from build123d import *

# Parameters (mm, degrees)
F0_R      = 5.334
F1_DEPTH  = 37.084
F2_R      = 2.032
F3_DEPTH  = 8.128
F4_W      = 3.0226
F4_H      = 47.752
F5_DEPTH  = 10.16
F7_DEPTH  = 3.0226
F9_DEPTH  = 3.0226
F10_R     = 2.54
F11_R     = 1.143
F13_DEPTH = 0.127


# Not quite as in the source:
# - a feature of the source that left no trace in its solid (it failed there, or was rolled back) is left out


with BuildPart() as f1:
    # F0 (on Top) → F1 (new body)
    with BuildSketch(Plane.XY):
        Circle(F0_R)
    extrude(amount=F1_DEPTH)

    # F2 (on Front) → F3 (join)
    with BuildSketch(Plane.XZ):
        with Locations((0, 6.2738)):
            Circle(F2_R)
    extrude(amount=-F3_DEPTH)

    # F4 (on face) → F5 (join, symmetric)
    with BuildSketch(Plane.XY.offset(37.084)):
        with Locations((0, 13.208)):
            Rectangle(F4_W, F4_H)
    extrude(amount=F5_DEPTH, both=True)

    # F6 (on face) → F7 (join)
    with BuildSketch(Plane(origin=(-1.5113, 0, 0), x_dir=(0, -1, 0), z_dir=(-1, 0, 0))):
        Polygon((15.748, 47.244), (10.668, 47.244), (10.668, 26.924), align=None)
        Polygon((-37.084, 47.244), (-37.084, 26.924), (-32.004, 47.244), align=None)
    extrude(amount=-F7_DEPTH)

    # F8 (on face) → F9 (cut, through all)
    with BuildSketch(Plane(origin=(-1.5113, 0, 0), x_dir=(0, -1, 0), z_dir=(-1, 0, 0))):
        Polygon((-37.084, 47.244), (-37.084, 26.924), (-32.004, 47.244), align=None)
    extrude(amount=-F9_DEPTH, mode=Mode.SUBTRACT)

    # F10
    f10_edges = [f1.edges().sort_by_distance(p)[0] for p in [
        (0, 32.004, 47.244),
        (0, 37.084, 26.924),
        (0, -15.748, 47.244),
        (0, -10.668, 26.924),
    ]]
    fillet(f10_edges, radius=F10_R)

    # F11
    f11_edges = [f1.edges().sort_by_distance(p)[0] for p in [
        (-1.5113, 8.763, 47.244),
        (1.5113, 8.763, 47.244),
        (-1.5113, 34.38999, 37.70004),
        (1.5113, 34.38999, 37.70004),
        (1.5113, 31.583975, 46.706042),
        (-1.5113, 31.583975, 46.706042),
        (-1.5113, 35.83287, 27.900853),
        (1.5113, 35.83287, 27.900853),
        (1.5113, 19.473124, 26.924),
        (-1.5113, 19.473124, 26.924),
        (1.5113, -14.49687, 46.267147),
        (1.5113, -13.05399, 36.46796),
        (-1.5113, -14.49687, 46.267147),
        (-1.5113, -13.05399, 36.46796),
        (1.5113, -10.247975, 27.461958),
        (1.5113, -6.900124, 26.924),
        (-1.5113, -6.900124, 26.924),
        (-1.5113, -10.247975, 27.461958),
    ]]
    fillet(f11_edges, radius=F11_R)

    # F12 (on face) → F13 (join)
    with BuildSketch(Plane.YZ.offset(1.5113)):
        with BuildLine():
            Line((-6.1186332318, 29.319293674), (-9.2636532318, 29.319293674))
            ThreePointArc((-9.2636532318, 29.319293674), (-9.0520071402, 28.9937255277), (-8.6848279277, 28.8673605332))
            Line((-8.6848279277, 28.8673605332), (-5.9157811718, 28.8673605332))
            Line((-5.9157811718, 28.8673605332), (-6.1186332318, 29.319293674))
        make_face()
        Polygon((-9.9286332318, 44.559293674), (-13.0736532318, 44.559293674), (-9.2636532318, 29.319293674), (-6.1186332318, 29.319293674), align=None)
        Polygon((-3.6385932318, 44.559293674), (-6.7836132318, 44.559293674), (-5.1148799466, 37.8843605332), (-1.9698599466, 37.8843605332), align=None)
        Polygon((2.6514467682, 44.559293674), (-0.4935732318, 44.559293674), (1.1751600534, 37.8843605332), (4.3201800534, 37.8843605332), align=None)
        with BuildLine():
            ThreePointArc((33.8308279277, 28.8673605332), (34.3011024, 29.0968207875), (34.4096532318, 29.608706326))
            Line((34.4096532318, 29.608706326), (33.8308279277, 29.464))
            Line((33.8308279277, 29.464), (31.6216067682, 29.319293674))
            Line((31.6216067682, 29.319293674), (28.4765867682, 29.319293674))
            Line((28.4765867682, 29.319293674), (25.3315667682, 29.319293674))
            Line((25.3315667682, 29.319293674), (22.1865467682, 29.319293674))
            Line((22.1865467682, 29.319293674), (19.0415267682, 29.319293674))
            Line((19.0415267682, 29.319293674), (15.8965067682, 29.319293674))
            Line((15.8965067682, 29.319293674), (12.7514867682, 29.319293674))
            Line((12.7514867682, 29.319293674), (9.6064667682, 29.319293674))
            Line((9.6064667682, 29.319293674), (6.4614467682, 29.319293674))
            Line((6.4614467682, 29.319293674), (5.9157811718, 31.5019560598))
            Line((5.9157811718, 31.5019560598), (5.9157811718, 28.8673605332))
            Line((5.9157811718, 28.8673605332), (33.8308279277, 28.8673605332))
        make_face()
        with BuildLine():
            ThreePointArc((-12.4948279277, 45.3006394668), (-12.9651024, 45.0711792125), (-13.0736532318, 44.559293674))
            Line((-13.0736532318, 44.559293674), (-9.9286332318, 44.559293674))
            Line((-9.9286332318, 44.559293674), (-6.7836132318, 44.559293674))
            Line((-6.7836132318, 44.559293674), (-3.6385932318, 44.559293674))
            Line((-3.6385932318, 44.559293674), (-0.4935732318, 44.559293674))
            Line((-0.4935732318, 44.559293674), (2.6514467682, 44.559293674))
            Line((2.6514467682, 44.559293674), (5.7964667682, 44.559293674))
            Line((5.7964667682, 44.559293674), (8.9414867682, 44.559293674))
            Line((8.9414867682, 44.559293674), (12.0865067682, 44.559293674))
            Line((12.0865067682, 44.559293674), (15.2315267682, 44.559293674))
            Line((15.2315267682, 44.559293674), (18.3765467682, 44.559293674))
            Line((18.3765467682, 44.559293674), (21.5215667682, 44.559293674))
            Line((21.5215667682, 44.559293674), (24.6665867682, 44.559293674))
            Line((24.6665867682, 44.559293674), (27.8116067682, 44.559293674))
            Line((27.8116067682, 44.559293674), (30.6720063948, 44.559293674))
            Line((30.6720063948, 44.559293674), (30.5996532318, 44.848706326))
            ThreePointArc((30.5996532318, 44.848706326), (30.3880071402, 45.1742744723), (30.0208279277, 45.3006394668))
            Line((30.0208279277, 45.3006394668), (-12.4948279277, 45.3006394668))
        make_face()
        Polygon((8.9414867682, 44.559293674), (5.7964667682, 44.559293674), (9.6064667682, 29.319293674), (12.7514867682, 29.319293674), align=None)
        Polygon((15.2315267682, 44.559293674), (12.0865067682, 44.559293674), (15.8965067682, 29.319293674), (19.0415267682, 29.319293674), align=None)
        Polygon((25.3315667682, 29.319293674), (21.5215667682, 44.559293674), (18.3765467682, 44.559293674), (22.1865467682, 29.319293674), align=None)
        Polygon((31.6216067682, 29.319293674), (27.8116067682, 44.559293674), (24.6665867682, 44.559293674), (28.4765867682, 29.319293674), align=None)
    extrude(amount=F13_DEPTH)

    # F14: F1 across plane


with BuildPart() as f1_1:
    add(f1.part)
    add(f1.part.mirror(Plane.YZ))

    # F17: F1 across plane


with BuildPart() as f1_2:
    add(f1_1.part)
    add(f1_1.part.mirror(Plane.YZ))


solid = f1_2.part
Could you check a few things on this model? Use its own coordinates, in mm. A direction names the side the tool comes from. Round coordinates to 2 decimals unless told otherwise and drop trailing zeros. Order: outer loops, then holes, each group sorted by start corner. A loop starts at its lowest first (then second) coordinate and runs counter-clockwise, first axis right, second up. Notation, with made-up numbers: M -1.75,-7 L 38.25,-7 A26 ccw 38.25,22 Z; hole C 6,35 d2. An arc over 180 degrees is marked long. One line per item, written item: value.
(1) Imagine slicing it at C-C (y = -4.5). Write out the boundary of the cut face in (x, z), and give its area (3 significant figures).
Ans:
outline: M -2.86,0 L 2.86,0 L 2.86,37.08 L 1.51,37.08 L 1.51,37.88 L 1.64,37.88 L 1.64,45.3 L 1.51,45.3 L 1.51,46.1 A1.14 ccw 0.37,47.24 L -0.37,47.24 A1.14 ccw -1.51,46.1 L -1.51,45.3 L -1.64,45.3 L -1.64,37.88 L -1.51,37.88 L -1.51,37.08 L -2.86,37.08 Z
area: 244 mm^2
(2) Imagine slicing it at D-D (x = -4.25). Write out the boundary of the cut face in (y, z), and give its area (3 significant figures).
Ans:
outline: M -3.22,0 L 3.22,0 L 3.22,37.08 L -3.22,37.08 Z
area: 239 mm^2
(3) Imagine slicing it at A-A (y = 27). Write out the boundary of the cut face in (x, z), and give its area (3 significant figures).
Ans:
outline: M -1.64,28.87 L -1.51,28.87 L -1.51,28.07 A1.14 ccw -0.37,26.92 L 0.37,26.92 A1.14 ccw 1.51,28.07 L 1.51,28.87 L 1.64,28.87 L 1.64,29.32 L 1.51,29.32 L 1.51,35.23 L 1.64,35.23 L 1.64,45.3 L 1.51,45.3 L 1.51,46.1 A1.14 ccw 0.37,47.24 L -0.37,47.24 A1.14 ccw -1.51,46.1 L -1.51,45.3 L -1.64,45.3 L -1.64,35.23 L -1.51,35.23 L -1.51,29.32 L -1.64,29.32 Z
area: 63.0 mm^2
(4) I need wall thicknesses on line 1 along Z through (x, y) = (0.5, 3); line 2 along X through (y, z) = (19.5, 30); line 3 along Z through (x, y) = (2.5, 4). Which ranges of each line are inside material? Lowest first, please. Write a range as from..to.
Ans:
line 1: z = 0..47.24
line 2: x = -1.51..1.51
line 3: z = 0..37.08
(5) If we mould it in two halves opening along Z, with no side actions, what happens to faces 1 (the flat face through (1.511, 12, 37)), 2 (the flat face through (-1.638, 10, 37)), 3 (the flat face through (-1.511, 12, 37)), 4 (the cylindrical face through (0.005, 35.853, 27.926))? For each: released by +Z, released by -Z, zero draft, split by the parting line, or undercut.
Ans:
face 1: undercut
face 2: zero draft
face 3: undercut
face 4: split by the parting line
(6) I'm going to push flat-ended pins straight in: P1, Ø12, axis at y = 24, z = 21.5, coming from the +X side; P2, Ø3.5, axis at x = -0.5, z = 7, coming from the +Y side; P3, Ø12, axis at y = 9.5, z = 9.5, coming from the +X side; P4, Ø12, axis at y = 17, z = 16, coming from the +X side. Where does each tip first touch, or does it pass through?
Ans:
P1: stops at x = 1.36
P2: stops at y = 8.13
P3: stops at x = 4.03
P4: passes through
(7) Imagine slicing it at B-B (z = 23). Write out the boundary of the cut face in (x, y), and give its area (3 significant figures).
Ans:
outline: C 0,0 d10.67
area: 89.4 mm^2
(8) Which directions (+Z, -Z, +X, -X, +Y, -Y) give clear straight access to the entire face, cutting with the end or side of a thin tool? Please do faces 5 (the cylindrical face through (1.17, -6.93, 27.25)), 6 (the cylindrical face through (0.01, -10.27, 27.48)).
Ans:
face 5: -Z, +X, -Y
face 6: -Z, +X, -X, -Y
